Here's how the part is built. I have some questions about the finished solid (model axes, mm). A direction names the side the tool comes from. Coordinates: 2 decimals unless noted, no trailing zeros. Loops run counter-clockwise (first coordinate to the right, second up) from the corner with the lowest first, then second, coordinate; pieces in that order, holes last. Notation, with made-up numbers: (39.25, -15) -> (86.25, -15) arc R27 ccw to (86.25, 7) -> close; hole circle Ø10 at (34.25, -6.75). An arc over 180 degrees is marked (long way). Answer as a JSON object with one key per item and string values. Group by question number.
1) I want a section at C-C (y = 8). Write out the boundary of the cut face in (x, z), then the cut area to 3 significant figures.
2) I need wall thicknesses on probe 1 along X at (y, z) = (1.5, 6.35); probe 2 along Y at (x, z) = (-13, 12); probe 3 along Y at (x, z) = (0, 9). Which ranges of each line are inside material? Lowest first, please. Write a range as [from, to].
3) I want a section at D-D (x = 0). Write out the boundary of the cut face in (y, z).
4) I want a section at B-B (z = 4.25). Write out the boundary of the cut face in (x, y).
5) Which directions (+Z, -Z, +X, -X, +Y, -Y) give clear straight access to the entire face, cutting with the end or side of a thin tool? Please do faces 1 (the flat face through (-12.7, 9, 6)), 2 (the flat face through (18, 6.35, 3)), 3 (the cylindrical face through (-1.39, 6.44, 6.26)).
6) I'm going to push flat-ended pins straight in: pin 1 (1.4 mm diameter, centred on x = 0, z = 6.35, fed in from +Y); pin 2 (4 mm diameter, centred on y = 13, z = 6.5, fed in from -X); pin 3 (5 mm diameter, centred on y = 18.5, z = 7, fed in from -X). Where does each tip first touch, or does it pass through?
7) If we mould it in two halves opening along X, with no side actions, what happens to faces 4 (the flat face through (0, 4, 0)), 5 (the cylindrical face through (0.245, 22.161, 7.453)), 6 (the flat face through (12.7, 10, 6))? For each: +X half, -X half, draft (parallel to the pull), parting line (faces both ways), or undercut.
8) I want a section at A-A (x = -19.05). Write out the boundary of the cut face in (y, z), then the cut area to 3 significant figures.
```python
from build123d import *

# Parameters (mm, degrees)
SKETCH1_R                 = 6.4135
BOSS_EXTRUDE1_DEPTH       = 12.7
SKETCH2_R                 = 3.2639
CUT_EXTRUDE1_DEPTH        = 7.35
F_4_40_TAPPED_HOLE1_D     = 2.2606
F_4_40_TAPPED_HOLE1_DEPTH = 7.62
F_4_40_TAPPED_HOLE1_TIP   = 0.679152758


with BuildPart() as part:
    # Sketch1 → Boss-Extrude1 (new body)
    with BuildSketch(Plane.XY):
        with BuildLine():
            Line((12.7, 12.7), (12.7, 6.35))
            Line((12.7, 6.35), (25.4, 6.35))
            Line((25.4, 6.35), (25.4, 0))
            Line((25.4, 0), (-25.4, 0))
            Line((-25.4, 0), (-25.4, 6.35))
            Line((-25.4, 6.35), (-12.7, 6.35))
            Line((-12.7, 6.35), (-12.7, 12.7))
            ThreePointArc((-12.7, 12.7), (0, 25.4), (12.7, 12.7))
        make_face()
        with Locations((0, 12.7)):
            Circle(SKETCH1_R, mode=Mode.SUBTRACT)
    extrude(amount=BOSS_EXTRUDE1_DEPTH)

    # Sketch2 → Cut-Extrude1 (cut, through all)
    with BuildSketch(Plane(origin=(0, 6.35, 0), x_dir=(1, 0, 0), z_dir=(0, 1, 0))):
        with Locations((19.05, -6.35)):
            Circle(SKETCH2_R)
        with Locations((-19.05, -6.35)):
            Circle(SKETCH2_R)
    extrude(amount=-CUT_EXTRUDE1_DEPTH, mode=Mode.SUBTRACT)

    # #4-40 Tapped Hole1
    with Locations(Plane(origin=(0, 25.4, 6.35), x_dir=(1, 0, 0), z_dir=(0, 1, 0))):
        with Locations((0, 0)):
            Hole(F_4_40_TAPPED_HOLE1_D / 2, depth=F_4_40_TAPPED_HOLE1_DEPTH)
            with Locations((0, 0, -(F_4_40_TAPPED_HOLE1_DEPTH + F_4_40_TAPPED_HOLE1_TIP / 2))):  # 118° drill point
                Cone(0, F_4_40_TAPPED_HOLE1_D / 2, F_4_40_TAPPED_HOLE1_TIP, mode=Mode.SUBTRACT)


solid = part.part
```
Determined:
{
 "1": {"outline": "(-12.7, 0) -> (-4.36, 0) -> (-4.36, 12.7) -> (-12.7, 12.7) -> close; (4.36, 0) -> (12.7, 0) -> (12.7, 12.7) -> (4.36, 12.7) -> close", "area": "212 mm^2"},
 "2": {"probe 1": "[-25.4, -22.31], [-15.79, 15.79], [22.31, 25.4]", "probe 2": "[0, 6.35]", "probe 3": "[0, 6.29], [19.11, 25.4]"},
 "3": {"outline": "(0, 0) -> (6.29, 0) -> (6.29, 12.7) -> (0, 12.7) -> close; (19.11, 0) -> (25.4, 0) -> (25.4, 5.22) -> (19.11, 5.22) -> close; (19.11, 7.48) -> (25.4, 7.48) -> (25.4, 12.7) -> (19.11, 12.7) -> close"},
 "4": {"outline": "(-25.4, 0) -> (-21.55, 0) -> (-21.55, 6.35) -> (-25.4, 6.35) -> close; (-16.55, 0) -> (16.55, 0) -> (16.55, 6.35) -> (12.7, 6.35) -> (12.7, 12.7) arc R12.7 ccw to (-12.7, 12.7) -> (-12.7, 6.35) -> (-16.55, 6.35) -> close; (21.55, 0) -> (25.4, 0) -> (25.4, 6.35) -> (21.55, 6.35) -> close; hole circle Ø12.83 at (0, 12.7)"},
 "5": {"face 1": "+Z, -Z, -X, +Y", "face 2": "+Z, -Z, +X, +Y", "face 3": "+Z, -Z"},
 "6": {"pin 1": "y = 6.32", "pin 2": "x = -12.7", "pin 3": "x = -12.26"},
 "7": {"face 4": "draft", "face 5": "undercut", "face 6": "+X half"},
 "8": {"outline": "(0, 0) -> (6.35, 0) -> (6.35, 3.09) -> (0, 3.09) -> close; (0, 9.61) -> (6.35, 9.61) -> (6.35, 12.7) -> (0, 12.7) -> close", "area": "39.2 mm^2"}
}
